Check sheet for the drawn part. Datum: minimum x, y, z corner. Units: mm. A direction names the side the tool comes from. Give positions to 0.01 mm unless a question says otherwise; leave off trailing zeros. Loops run counter-clockwise (first coordinate to the right, second up) from the corner with the lowest first, then second, coordinate; pieces in that order, holes last. Notation, with made-up numbers: M -20.75,23.5 L -3.75,23.5 A12 ccw -3.75,30.5 Z; hole C 67.25,-14 d10. An arc over 180 degrees is marked long. Write each question's results on one line, items separated by ' | '. Start each with the question number.
1. Tool access check on the marked faces 1 and 2. Record the directions out of +Z, -Z, +X, -X, +Y, -Y that give a thin tool (end or side, any length) a straight path to the whole face; none if there is none.
2. Sectioned sample at B-B on x = 33. Record the cut outline in (y, z).
3. Sectioned sample at A-A on z = 30.5. Record the cut outline in (x, y).
4. Sectioned sample at D-D on y = 5.75. Record the cut outline in (x, z), and give its area (3 significant figures).
5. Sectioned sample at C-C on x = 43.5. Record the cut outline in (y, z), and give its area (3 significant figures).
6. Material ranges on line 1 along X through (y, z) = (4.25, 6); line 2 along Z through (x, y) = (35, 5); line 3 along Y through (x, z) = (12, 39), recorded low to high.
7. Go/stop test with flat-tipped pins: pin 1 (6 mm diameter, centred on y = 13, z = 18, fed in from -X); pin 2 (10 mm diameter, centred on x = 26.5, z = 22.5, fed in from -Y); pin 3 (1.5 mm diameter, centred on x = 37.5, z = 19, fed in from -Y). Record where each tip stops, or that it passes through.
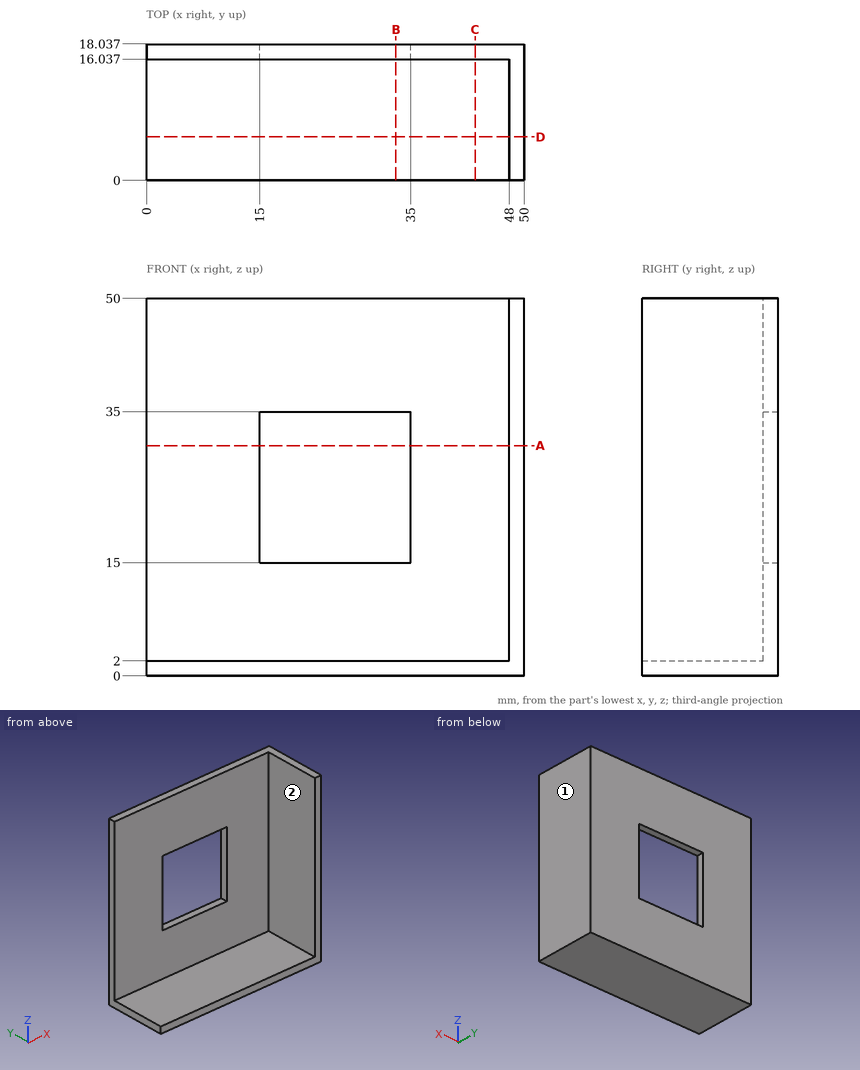
Output values:
1) face 1: +Z, -Z, +X, +Y, -Y | face 2: +Z, -X, -Y
2) outline: M 0,0 L 18.04,0 L 18.04,15 L 16.04,15 L 16.04,2 L 0,2 Z; M 16.04,35 L 18.04,35 L 18.04,50 L 16.04,50 Z
3) outline: M 0,16.04 L 15,16.04 L 15,18.04 L 0,18.04 Z; M 35,16.04 L 48,16.04 L 48,0 L 50,0 L 50,18.04 L 35,18.04 Z
4) outline: M 0,0 L 50,0 L 50,50 L 48,50 L 48,2 L 0,2 Z | area: 196 mm2
5) outline: M 0,0 L 18.04,0 L 18.04,50 L 16.04,50 L 16.04,2 L 0,2 Z | area: 132 mm2
6) line 1: 48 to 50 | line 2: 0 to 2 | line 3: 16.04 to 18.04
7) pin 1: x = 48 | pin 2: through | pin 3: y = 16.04
